```python
from build123d import *

# Parameters (mm, degrees)
F0_W     = 88.9
F0_H     = 50.8
F1_DEPTH = 3.2
F2_R     = 2.54
F4_W     = 3.3
F4_H     = 3.3
F5_DEPTH = 2
F7_W     = 2
F7_H     = 2
F8_DEPTH = 1.5


with BuildPart() as f1:
    # F0 (on Top) → F1 (new body)
    with BuildSketch(Plane.XY):
        Rectangle(F0_W, F0_H)
    extrude(amount=F1_DEPTH)

    # F2
    f2_edges = [f1.edges().sort_by_distance(p)[0] for p in [
        (44.45, -25.4, 1.6),
        (44.45, 25.4, 1.6),
        (-44.45, -25.4, 1.6),
        (-44.45, 25.4, 1.6),
    ]]
    fillet(f2_edges, radius=F2_R)

    # F4 (on face) → F5 (join)
    with BuildSketch(Plane(origin=(0, 0, 0), x_dir=(1, 0, 0), z_dir=(0, 0, -1))):
        with Locations((25.4, 0)):
            Rectangle(F4_W, F4_H)
    extrude(amount=F5_DEPTH)

    # F7 (on face) → F8 (join)
    with BuildSketch(Plane(origin=(0, 0, 0), x_dir=(1, 0, 0), z_dir=(0, 0, -1))):
        with Locations((20.4, 0)):
            Rectangle(F7_W, F7_H)
    extrude(amount=F8_DEPTH)


solid = f1.part
```
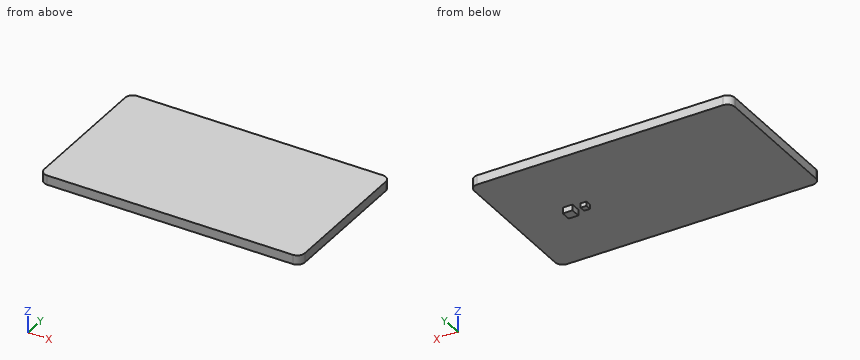
Input: part model. Units: mm. Frame: model coordinates. Round coordinates to 2 decimals unless told otherwise and drop trailing zeros. Write each loop counter-clockwise with the first axis right and the second up, starting at its lowest first coordinate (ties: lowest second). Pieces come first, ordered by that corner, then holes. Notation, with made-up numbers: (8.25, -3.75) -> (45.25, -3.75) arc R24 cw to (45.25, 28.25) -> close; hole circle Ø4 at (-20, 1.25). An arc over 180 degrees is marked (long way). Answer as CSV lines item,"result".
1. Contact query for flat-ended pins moving along their axis: P1, Ø3, axis at x = 18.5, y = 5.5, coming from the -Z side; P2, Ø1, axis at y = 0.5, z = -1, coming from the +X side; P3, Ø1.6, axis at x = 25, z = -1, coming from the -Y side; P4, Ø1, axis at x = -17, z = -1, coming from the -Y side. Output: stop coordinate, or through.
Geometry says:
P1,"stops at z = 0"
P2,"stops at x = 27.05"
P3,"stops at y = -1.65"
P4,"passes through"
2. Section A-A (x = -28.5). Return the cut outline in (y, z).
Geometry says:
outline,"(-25.4, 0) -> (25.4, 0) -> (25.4, 3.2) -> (-25.4, 3.2) -> close"
3. Section B-B (y = -6). Return the cut outline in (x, z), plus the area to 3 significant figures.
Geometry says:
outline,"(-44.45, 0) -> (44.45, 0) -> (44.45, 3.2) -> (-44.45, 3.2) -> close"
area,"284 mm^2"
4. Ray query, L1, parallel to Z at x = -1.5, y = -15; L2, parallel to Y at x = 26, z = -0.45. Return the intervals inside material, ascending. Write a range as [from, to].
Geometry says:
L1,"z = [0, 3.2]"
L2,"y = [-1.65, 1.65]"
